from build123d import *

# Parameters (mm, degrees)
F1_DEPTH = 25.4


with BuildPart() as f1:
    # F0 (on Top) → F1 (new body)
    with BuildSketch(Plane.XY):
        with BuildLine():
            Line((63.499014, 0), (76.2, 0))
            ThreePointArc((76.2, 0), (75.933086, 6.372321), (75.134213, 12.7))
            Line((75.134213, 12.7), (62.216033, 12.7))
            ThreePointArc((62.216033, 12.7), (63.177455, 6.38232), (63.499014, 0))
        make_face()
        with BuildLine():
            ThreePointArc((75.134213, -12.7), (75.933086, -6.372321), (76.2, 0))
            Line((76.2, 0), (63.499014, 0))
            ThreePointArc((63.499014, 0), (63.177455, -6.38232), (62.216033, -12.7))
            Line((62.216033, -12.7), (75.134213, -12.7))
        make_face()
        with BuildLine():
            Line((62.216033, 12.7), (75.134213, 12.7))
            ThreePointArc((75.134213, 12.7), (53.881537, 53.881537), (12.7, 75.134213))
            Line((12.7, 75.134213), (12.7, 62.216033))
            ThreePointArc((12.7, 62.216033), (44.900584, 44.900584), (62.216033, 12.7))
        make_face()
        with BuildLine():
            ThreePointArc((12.7, -75.134213), (53.881537, -53.881537), (75.134213, -12.7))
            Line((75.134213, -12.7), (62.216033, -12.7))
            ThreePointArc((62.216033, -12.7), (44.900584, -44.900584), (12.7, -62.216033))
            Line((12.7, -62.216033), (12.7, -75.134213))
        make_face()
        with BuildLine():
            Line((12.7, 62.216033), (12.7, 75.134213))
            ThreePointArc((12.7, 75.134213), (6.372321, 75.933086), (0, 76.2))
            Line((0, 76.2), (0, 63.499014))
            ThreePointArc((0, 63.499014), (6.38232, 63.177455), (12.7, 62.216033))
        make_face()
        with BuildLine():
            ThreePointArc((0, -76.2), (6.372321, -75.933086), (12.7, -75.134213))
            Line((12.7, -75.134213), (12.7, -62.216033))
            ThreePointArc((12.7, -62.216033), (6.38232, -63.177455), (0, -63.499014))
            Line((0, -63.499014), (0, -76.2))
        make_face()
        with BuildLine():
            Line((0, 63.499014), (0, 76.2))
            ThreePointArc((0, 76.2), (-6.372321, 75.933086), (-12.7, 75.134213))
            Line((-12.7, 75.134213), (-12.7, 62.216033))
            ThreePointArc((-12.7, 62.216033), (-6.38232, 63.177455), (0, 63.499014))
        make_face()
        with BuildLine():
            ThreePointArc((-12.7, -75.134213), (-6.372321, -75.933086), (0, -76.2))
            Line((0, -76.2), (0, -63.499014))
            ThreePointArc((0, -63.499014), (-6.38232, -63.177455), (-12.7, -62.216033))
            Line((-12.7, -62.216033), (-12.7, -75.134213))
        make_face()
        with BuildLine():
            Line((-12.7, 62.216033), (-12.7, 75.134213))
            ThreePointArc((-12.7, 75.134213), (-53.881537, 53.881537), (-75.134213, 12.7))
            Line((-75.134213, 12.7), (-62.216033, 12.7))
            ThreePointArc((-62.216033, 12.7), (-44.900584, 44.900584), (-12.7, 62.216033))
        make_face()
        with BuildLine():
            ThreePointArc((-75.134213, -12.7), (-53.881537, -53.881537), (-12.7, -75.134213))
            Line((-12.7, -75.134213), (-12.7, -62.216033))
            ThreePointArc((-12.7, -62.216033), (-44.900584, -44.900584), (-62.216033, -12.7))
            Line((-62.216033, -12.7), (-75.134213, -12.7))
        make_face()
        with BuildLine():
            Line((-62.216033, 12.7), (-75.134213, 12.7))
            ThreePointArc((-75.134213, 12.7), (-75.933086, 6.372321), (-76.2, 0))
            Line((-76.2, 0), (-63.499014, 0))
            ThreePointArc((-63.499014, 0), (-63.177455, 6.38232), (-62.216033, 12.7))
        make_face()
        with BuildLine():
            ThreePointArc((-76.2, 0), (-75.933086, -6.372321), (-75.134213, -12.7))
            Line((-75.134213, -12.7), (-62.216033, -12.7))
            ThreePointArc((-62.216033, -12.7), (-63.177455, -6.38232), (-63.499014, 0))
            Line((-63.499014, 0), (-76.2, 0))
        make_face()
    extrude(amount=F1_DEPTH)


solid = f1.part
Here's how the part is built. I have some questions about the finished solid (model axes, mm). A direction names the side the tool comes from. Give positions to 0.01 mm unless a question says otherwise; leave off trailing zeros. Order: outer loops, then holes, each group sorted by start corner. A loop starts at its lowest first (then second) coordinate and runs counter-clockwise, first axis right, second up. Notation, with made-up numbers: (-7, 36) -> (25, 36) arc R19 ccw to (25, 69) -> close; hole circle Ø3 at (49, 16). An arc over 180 degrees is marked (long way). One line per item, written item: value. Start each with the question number.
1. For faces 1 (the face through (-44.5, -45.3, 12.5)), 2 (the face through (-29, 57, 0)), which set-ups out of +Z, -Z, +X, -X, +Y, -Y let a thin tool reach every point of the face, with its end or its side?
2. Imagine slicing it at A-A, the plane z = 13.5. List the corners of the cut face in (x, y) for me.
3. Imagine slicing it at B-B, the plane x = 42. List the corners of the cut face in (y, z) for me.
4. Imagine slicing it at C-C, the plane y = -59. List the corners of the cut face in (x, z) for me, plus the area to 3 significant figures.
5. Will these pins go through, and if not, where does the flat tip stop? pin 1 Ø5 at (y, z) = (-58, 17.5) entering from +X; pin 2 Ø1.5 at (y, z) = (27, 22.5) entering from -X; pin 3 Ø8 at (x, z) = (-47.5, 16.5) entering from -Y.
6. I need wall thicknesses on probe 1 along Y at (x, z) = (-12.5, 10.75); probe 2 along X at (y, z) = (-1, 8.5); probe 3 along Y at (x, z) = (-40, 8.75). Which ranges of each line are inside material? Lowest first, please. Write a range as from..to.
7. We'd pull the mould along Y, two halves only. Please class faces 3 (the face through (54.35, 53.41, 12.52)), 4 (the face through (-54.35, -53.41, 12.52)), 5 (the face through (45.3, -44.5, 12.5)): released by +Y, released by -Y, zero draft, split by the parting line, or undercut.
Values follow:
1. face 1: +Z, -Z
1. face 2: -Z, +X, -X, +Y, -Y
2. outline: (-76.2, 0) arc R76.2 ccw to (-75.13, -12.7) arc R76.2 ccw to (-12.7, -75.13) arc R76.2 ccw to (0, -76.2) arc R76.2 ccw to (12.7, -75.13) arc R76.2 ccw to (75.13, -12.7) arc R76.2 ccw to (76.2, 0) arc R76.2 ccw to (75.13, 12.7) arc R76.2 ccw to (12.7, 75.13) arc R76.2 ccw to (0, 76.2) arc R76.2 ccw to (-12.7, 75.13) arc R76.2 ccw to (-75.13, 12.7) arc R76.2 ccw to start; hole (-63.5, 0) arc R63.5 ccw to (-62.22, -12.7) arc R63.5 ccw to (-12.7, -62.22) arc R63.5 ccw to (0, -63.5) arc R63.5 ccw to (12.7, -62.22) arc R63.5 ccw to (62.22, -12.7) arc R63.5 ccw to (63.5, 0) arc R63.5 ccw to (62.22, 12.7) arc R63.5 ccw to (12.7, 62.22) arc R63.5 ccw to (0, 63.5) arc R63.5 ccw to (-12.7, 62.22) arc R63.5 ccw to (-62.22, 12.7) arc R63.5 ccw to start
3. outline: (-63.58, 0) -> (-47.62, 0) -> (-47.62, 25.4) -> (-63.58, 25.4) -> close; (47.62, 0) -> (63.58, 0) -> (63.58, 25.4) -> (47.62, 25.4) -> close
4. outline: (-48.22, 0) -> (-23.48, 0) -> (-23.48, 25.4) -> (-48.22, 25.4) -> close; (23.48, 0) -> (48.22, 0) -> (48.22, 25.4) -> (23.48, 25.4) -> close
4. area: 1,260 mm2
5. pin 1: stops at x = 52.21
5. pin 2: stops at x = -71.54
5. pin 3: stops at y = -62.56
6. probe 1: y = -75.17..-62.26, 62.26..75.17
6. probe 2: x = -76.19..-63.49, 63.49..76.19
6. probe 3: y = -64.86..-49.32, 49.32..64.86
7. face 3: released by +Y
7. face 4: released by -Y
7. face 5: undercut
